Part model, mm, in its own coordinate system. A direction names the side the tool comes from. Coordinates: 2 decimals unless noted, no trailing zeros. Order: outer loops, then holes, each group sorted by start corner. A loop starts at its lowest first (then second) coordinate and runs counter-clockwise, first axis right, second up. Notation, with made-up numbers: M 89,63 L 114,63 A32 cw 114,89 Z; hole C 59,3 d2. An arc over 180 degrees is marked long. Answer in a Markdown table with one row per item. Add a question column.
from build123d import *


with BuildPart() as f1:
    # F0 (on Front) → F1 (revolve)
    with BuildSketch(Plane.XZ):
        with BuildLine():
            Line((1, 0.85), (0, 0.85))
            Line((0, 0.85), (0, -0.75))
            Line((0, -0.75), (27, -0.75))
            Line((27, -0.75), (27, 0))
            Line((27, 0), (26.1339745962, 1.5))
            Line((26.1339745962, 1.5), (23.1180339887, 1.5))
            ThreePointArc((23.1180339887, 1.5), (22, 1), (20.8819660113, 1.5))
            Line((20.8819660113, 1.5), (2.09658561, 1.5))
            ThreePointArc((2.09658561, 1.5), (1.6373774392, 1.0247093416), (1, 0.85))
        make_face()
    revolve(axis=Axis((13.5, 0, -0.75), (-1, 0, 0)))

    # F5: sweep along a path in F4
    with BuildLine(Plane.XZ) as f5_path:
        Line((27, -2), (11.5, -2))
        ThreePointArc((11.5, -2), (10.4339207347, -2.2837767539), (9.65, -3.06))
    # F3 (on offset) → F5 (sweep, cut)
    with BuildSketch(Plane.YZ.offset(27)):
        Polygon((2.380318353, -2), (0, -2), (-2.619681647, -2), (-2.619681647, -3), (2.380318353, -3), align=None)
    sweep(path=f5_path.line, mode=Mode.SUBTRACT)


solid = f1.part
(1) Drop a flat-ended pin along its axis: P1, Ø1.9, axis at x = 21, y = -0.5, coming from the -Z side. Give the stop position or say it passes through.
(2) Wall check: line 1 (X direction, y = 0.55, z = 1.2); line 2 (X direction, y = 1.75, z = -1.7); line 3 (Y direction, x = 9.5, z = -2). Give the ranges that are in metal, low to high.
(3) Slice it at D-D (x = 2.5). List the corners of the cut face in (y, z).
(4) 3-axis set-ups, long thin cutter, end or side, ignore diameter. For faces 1 (the cylindrical face through (0.493, 0.481, 0.776)), 2 (the cylindrical face through (11.358, 0.676, 1.396)), 3 (the flat face through (19, 0, -2)): which of +Z, -Z, +X, -X, +Y, -Y reach the whole face in a straight line?
(5) Slice it at C-C (x = 19.25). List the corners of the cut face in (y, z), and give its area (3 significant figures).
(6) Slice it at A-A (z = -0.75). List the corners of the cut face in (x, y).
(7) Slice it at B-B (y = 0). List the corners of the cut face in (x, z), and give its area (3 significant figures).
Computed:
| question | item | result |
|---|---|---|
| 1 | P1 | stops at z = -2 |
| 2 | line 1 | x = 1.94 to 21.13, 22.87 to 26.26 |
| 2 | line 2 | x = 1.91 to 21.18, 22.82 to 26.28 |
| 2 | line 3 | y = -1.87 to 1.87 |
| 3 | outline | C 0,-0.75 d4.5 |
| 4 | face 1 | -X |
| 4 | face 2 | +X, -X |
| 4 | face 3 | -Z, +X, +Y, -Y |
| 5 | outline | M -1.87,-2 L 1.87,-2 A2.25 ccw long Z |
| 5 | area | 13.3 mm^2 |
| 6 | outline | M 0,-1.6 L 1,-1.6 A1.25 cw 2.1,-2.25 L 20.88,-2.25 A1.5 cw 23.12,-2.25 L 26.13,-2.25 L 27,-0.75 L 27,0.75 L 26.13,2.25 L 23.12,2.25 A1.5 cw 20.88,2.25 L 2.1,2.25 A1.25 cw 1,1.6 L 0,1.6 Z |
| 7 | outline | M 0,-2.35 L 1,-2.35 A1.25 cw 2.1,-3 L 9.69,-3 A2.14 cw 11.5,-2 L 26.71,-2 L 27,-1.5 L 27,0 L 26.13,1.5 L 23.12,1.5 A1.5 cw 20.88,1.5 L 2.1,1.5 A1.25 cw 1,0.85 L 0,0.85 Z |
| 7 | area | 101 mm^2 |
